For this review, take the finished solid that the model builds, in its own axes (mm). Give positions to 0.01 mm unless a question says otherwise; leave off trailing zeros. Loops run counter-clockwise (first coordinate to the right, second up) from the corner with the lowest first, then second, coordinate; pieces in that order, holes last. Notation, with made-up numbers: (-29.75, 38) - (26.25, 38) arc R13 ccw to (26.25, 59) - close; hole circle Ø7 at (53, 6). An arc over 180 degrees is marked (long way). Answer as CSV lines item,"result".
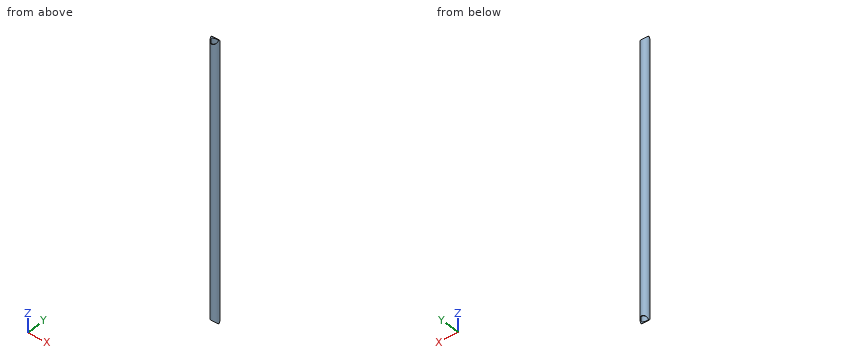
Autodesk Inventor part; units mm, degrees
ref_plane "作業平面1" through (0, 0, 0) normal (0, 1, 0) x (-1, 0, 0)
ref_plane "YZ Plane" through (0, 0, 0) normal (1, 0, 0) x (0, 1, 0)
ref_plane "XY Plane" through (0, 0, 0) normal (0, 0, 1) x (1, 0, 0)
sketch "スケッチ1" plane through (0, 0, 0) normal (0, 0, 1) x (1, 0, 0)
  circle A0 centre (0, 0) radius 13.6
  dimension "d0" = 27.2
extrude "押し出し1" add sketch "スケッチ1" against normal blind 1000
sketch "スケッチ3" plane through (0, 0, 0) normal (0, 0, 1) x (1, 0, 0)
  circle A0 centre (0, 0) radius 13.6
hole "穴1" at (0, 0, 0) direction (0, 0, -1) diameter 22.6 end through all
ref_plane "作業平面1" through (0, 0, 0) normal (0, 1, 0) x (-1, 0, 0)
sketch "スケッチ4" plane through (0, 0, 0) normal (0, 1, 0) x (-1, 0, 0)
  line L0 (-13.6, 0) -> (13.6, 0)
  arc A0 (-13.6, 0) -> (13.6, 0) centre (0, 0) ccw
  line L1 (13.6, 0) -> (-13.6, 0)
extrude "押し出し3" cut sketch "スケッチ4" along normal mid plane 27.2
sketch "スケッチ5" plane through (0, 0, 0) normal (0, 1, 0) x (-1, 0, 0)
  line L0 (-13.6, -1000) -> (13.6, -1000)
  arc A0 (13.6, -1000) -> (-13.6, -1000) centre (0, -1000) ccw
  line L1 (-13.6, -1000) -> (13.6, -1000)
  point P0 (0, 0)
extrude "押し出し4" cut sketch "スケッチ5" along normal mid plane 27.2
ref_plane "作業平面2" through (0, 0, 0) normal (0, 1, 0) x (-1, 0, 0)
properties part number "縦のパイプ"
1) Consider section C-C on z = -406. Write out the cut boundary in (x, y), and give its area (3 significant figures).
From the geometry:
outline,"circle Ø27.2 at (0, 0); hole circle Ø22.6 at (0, 0)"
area,"180 mm^2"
2) Insertion check: P1, Ø6, axis at x = -7, z = -802, coming from the -Y side; P2, Ø3, axis at y = 10, z = -688.5, coming from the +X side; P3, Ø6, axis at x = 9, y = 2, coming from the +Z side; P4, Ø5, axis at x = -6.5, y = -5.5, coming from the -Z side. Each pin has a flat end and moves straight along its axis. Give the tip position at first contact, or say it passes through.
From the geometry:
P1,"stops at y = -13"
P2,"stops at x = 10.62"
P3,"stops at z = -6.4"
P4,"passes through"
3) Consider section A-A on y = 0. Write out the cut boundary in (x, z), and give its area (3 significant figures).
From the geometry:
outline,"(-13.6, -1000) arc R13.6 cw to (-11.3, -992.43) - (-11.3, -7.57) arc R13.6 cw to (-13.6, 0) - close; (11.3, -992.43) arc R13.6 cw to (13.6, -1000) - (13.6, 0) arc R13.6 cw to (11.3, -7.57) - close"
area,"4,550 mm^2"
4) Consider section B-B on x = 7. Write out the cut boundary in (y, z).
From the geometry:
outline,"(-11.66, -988.34) - (-8.87, -988.34) - (-8.87, -11.66) - (-11.66, -11.66) - close; (8.87, -988.34) - (11.66, -988.34) - (11.66, -11.66) - (8.87, -11.66) - close"
5) Wall thickness on line 1 (X direction, y = 0, z = -772); line 2 (X direction, y = 1.75, z = -591.5); line 3 (Y direction, x = -6.5, z = -150.5): over which ranges is each line inside the solid? List them lowest first. Write a range as from..to.
From the geometry:
line 1,"x = -13.6..-11.3, 11.3..13.6"
line 2,"x = -13.49..-11.16, 11.16..13.49"
line 3,"y = -11.95..-9.24, 9.24..11.95"
